CAD build for the part. Positions are in the model's coordinates, mm. Coordinates: 2 decimals unless noted, no trailing zeros.
1) Saw through at A-A, the plane z = -5. Give the number of separate pieces and of enclosed holes in the cut face, and give its area (3 significant figures).
2) Wall check: line 1 along Y through (x, z) = (0, -11); line 2 along X through (y, z) = (52.5, -1); line 3 along Z through (x, y) = (66.5, 3). Give the ranges that are in metal, low to high.
3) Pin check, flat tips, straight feed: pin 1 Ø1 at (x, z) = (14.5, -12.5) entering from -Y; pin 2 Ø5 at (y, z) = (-6, -10) entering from +X; pin 3 Ø3 at (x, z) = (46, -1) entering from -Y; pin 4 Ø11 at (x, y) = (0, 0) entering from +Z. Stop position of each tip, or through.
```python
from build123d import *

# Parameters (mm, degrees)
CUT_EXTRUDE1_DEPTH      = 117.550418275
CUT_EXTRUDE1_DEPTH_BACK = 117.550418275


with BuildPart() as part:
    # Sketch1 → Revolve1 (revolve)
    with BuildSketch(Plane(origin=(0, 0, 0), x_dir=(0, 0, -1), z_dir=(1, 0, 0)), mode=Mode.PRIVATE) as revolve1_sk:
        Polygon((-14, 80), (14, 80), (14, 65), (10, 65), (10, 13), (18, 13), (18, 6), (-18, 6), (-18, 13), (-10, 13), (-10, 65), (-14, 65), align=None)
    revolve(revolve1_sk.sketch.rotate(Axis((0, 0, 21.009226083), (0, 0, -1)), 90), axis=Axis((0, 0, 21.009226083), (0, 0, -1)))

    # Sketch2 → Cut-Extrude1 (cut, two sides: drawn at the far end of the back side and taken through both)
    with BuildSketch(Plane(origin=(0, 0, -10), x_dir=(-1, 0, 0), z_dir=(0, 0, -1)).offset(-CUT_EXTRUDE1_DEPTH_BACK)):
        with BuildLine():
            Line((0.637719681, 16.747637536), (7.842487003, 59.087331998))
            ThreePointArc((7.842487003, 59.087331998), (7.789998599, 59.614078882), (7.47597205, 60.040229838))
            ThreePointArc((7.47597205, 60.040229838), (-4.486988844, 63.647600818), (-15.699134285, 58.13277051))
            ThreePointArc((-15.699134285, 58.13277051), (-15.940556782, 57.654586316), (-15.900550292, 57.120409916))
            Line((-15.900550292, 57.120409916), (-1.288879604, 16.576347699))
            ThreePointArc((-1.288879604, 16.576347699), (-0.259550601, 15.919320899), (0.637719681, 16.747637536))
        make_face()
        with BuildLine():
            Line((7.394463789, 15.040344235), (31.197451444, 50.789136914))
            ThreePointArc((31.197451444, 50.789136914), (31.36374816, 51.291693094), (31.250201842, 51.80872747))
            ThreePointArc((31.250201842, 51.80872747), (21.78874322, 59.969999397), (9.302855115, 59.492341617))
            ThreePointArc((9.302855115, 59.492341617), (8.887809655, 59.153693995), (8.707088287, 58.649427466))
            Line((8.707088287, 58.649427466), (5.56475791, 15.667481708))
            ThreePointArc((5.56475791, 15.667481708), (6.23785987, 14.648592036), (7.394463789, 15.040344235))
        make_face()
        with BuildLine():
            Line((12.872637931, 10.732438778), (49.15809311, 33.709038652))
            ThreePointArc((49.15809311, 33.709038652), (49.514420733, 34.1005076), (49.620987836, 34.619025454))
            ThreePointArc((49.620987836, 34.619025454), (44.297003636, 45.92304027), (32.696296351, 50.565146389))
            ThreePointArc((32.696296351, 50.565146389), (32.17939306, 50.424590588), (31.809192199, 50.037426194))
            Line((31.809192199, 50.037426194), (11.456198227, 12.049565795))
            ThreePointArc((11.456198227, 12.049565795), (11.6566877, 10.844988532), (12.872637931, 10.732438778))
        make_face()
        with BuildLine():
            Line((16.12501603, 4.568797156), (58.618853889, 10.800341371))
            ThreePointArc((58.618853889, 10.800341371), (59.103600137, 11.013034549), (59.411854241, 11.443379433))
            ThreePointArc((59.411854241, 11.443379433), (59.145909698, 23.935570282), (50.436250912, 32.894777979))
            ThreePointArc((50.436250912, 32.894777979), (49.906867064, 32.976617376), (49.411197804, 32.773499358))
            Line((49.411197804, 32.773499358), (15.366757794, 6.348170489))
            ThreePointArc((15.366757794, 6.348170489), (15.05996833, 5.166187987), (16.12501603, 4.568797156))
        make_face()
        with BuildLine():
            Line((16.589232367, -2.384831001), (57.943882296, -13.975833051))
            ThreePointArc((57.943882296, -13.975833051), (58.473230137, -13.978692226), (58.929871308, -13.710930852))
            ThreePointArc((58.929871308, -13.710930852), (63.767950649, -2.190577255), (59.455319492, 9.536603618))
            ThreePointArc((59.455319492, 9.536603618), (59.004990363, 9.826687436), (58.469558421, 9.842736744))
            Line((58.469558421, 9.842736744), (16.620265336, -0.450881165))
            ThreePointArc((16.620265336, -0.450881165), (15.859243619, -1.405893394), (16.589232367, -2.384831001))
        make_face()
        with BuildLine():
            Line((14.185019719, -8.926100213), (47.24988705, -36.335458973))
            ThreePointArc((47.24988705, -36.335458973), (47.732307435, -36.553376123), (48.258378264, -36.494496632))
            ThreePointArc((48.258378264, -36.494496632), (57.36393362, -27.937954084), (58.194023196, -15.470536147))
            ThreePointArc((58.194023196, -15.470536147), (57.900614785, -15.022366034), (57.418001208, -14.789924471))
            Line((57.418001208, -14.789924471), (14.999978011, -7.17197137))
            ThreePointArc((14.999978011, -7.17197137), (13.91631161, -7.734883035), (14.185019719, -8.926100213))
        make_face()
        with BuildLine():
            Line((9.328088295, -13.923965606), (28.385957082, -52.412353941))
            ThreePointArc((28.385957082, -52.412353941), (28.738035143, -52.807649211), (29.242573206, -52.967832403))
            ThreePointArc((29.242573206, -52.967832403), (41.041171333, -48.854604843), (46.870451614, -37.802679666))
            ThreePointArc((46.870451614, -37.802679666), (46.7846969, -37.273915943), (46.43834996, -36.865273382))
            Line((46.43834996, -36.865273382), (10.786058217, -12.65296257))
            ThreePointArc((10.786058217, -12.65296257), (9.567122898, -12.726441131), (9.328088295, -13.923965606))
        make_face()
        with BuildLine():
            Line((2.858245661, -16.514250851), (4.613837255, -59.426676761))
            ThreePointArc((4.613837255, -59.426676761), (4.774695497, -59.931000008), (5.170461579, -60.282548753))
            ThreePointArc((5.170461579, -60.282548753), (17.622017675, -61.323850595), (27.442553143, -53.598396444))
            ThreePointArc((27.442553143, -53.598396444), (27.579279895, -53.080467163), (27.429086125, -52.566281616))
            Line((27.429086125, -52.566281616), (4.70713097, -15.946141593))
            ThreePointArc((4.70713097, -15.946141593), (3.563691723, -15.517481939), (2.858245661, -16.514250851))
        make_face()
        with BuildLine():
            Line((-4.105813613, -16.249072097), (-19.956056948, -56.165587294))
            ThreePointArc((-19.956056948, -56.165587294), (-20.014232376, -56.691736448), (-19.795669826, -57.173864775))
            ThreePointArc((-19.795669826, -57.173864775), (-8.84414293, -63.189645469), (3.269587926, -60.126463551))
            ThreePointArc((3.269587926, -60.126463551), (3.605154846, -59.708923389), (3.677084113, -59.178102208))
            Line((3.677084113, -59.178102208), (-2.185701986, -16.482087868))
            ThreePointArc((-2.185701986, -16.482087868), (-3.055934127, -15.625409147), (-4.105813613, -16.249072097))
        make_face()
        with BuildLine():
            Line((-10.359940414, -13.174281159), (-41.07536761, -43.192957537))
            ThreePointArc((-41.07536761, -43.192957537), (-41.342517649, -43.649956627), (-41.338950081, -44.179300168))
            ThreePointArc((-41.338950081, -44.179300168), (-33.781070876, -54.129376582), (-21.468718747, -56.258118879))
            ThreePointArc((-21.468718747, -56.258118879), (-20.992334227, -56.013164323), (-20.710719147, -55.557491313))
            Line((-20.710719147, -55.557491313), (-8.700607211, -14.168131416))
            ThreePointArc((-8.700607211, -14.168131416), (-9.147161204, -13.031561162), (-10.359940414, -13.174281159))
        make_face()
        with BuildLine():
            Line((-14.8227394, -7.821537324), (-55.092374054, -22.751873025))
            ThreePointArc((-55.092374054, -22.751873025), (-55.522306034, -23.060702758), (-55.734350314, -23.545733206))
            ThreePointArc((-55.734350314, -23.545733206), (-52.876944776, -35.709646734), (-42.494888911, -42.662234363))
            ThreePointArc((-42.494888911, -42.662234363), (-41.960058003, -42.632220281), (-41.517450915, -42.330485445))
            Line((-41.517450915, -42.330485445), (-13.711098407, -9.404376329))
            ThreePointArc((-13.711098407, -9.404376329), (-13.656761009, -8.184437864), (-14.8227394, -7.821537324))
        make_face()
        with BuildLine():
            Line((-16.722552084, -1.116378629), (-59.583408526, 1.623217027))
            ThreePointArc((-59.583408526, 1.623217027), (-60.101783302, 1.515956117), (-60.492775047, 1.159104933))
            ThreePointArc((-60.492775047, 1.159104933), (-62.829914552, -11.115394554), (-56.173306729, -21.689661952))
            ThreePointArc((-56.173306729, -21.689661952), (-55.672506555, -21.879778052), (-55.145438246, -21.784154084))
            Line((-55.145438246, -21.784154084), (-16.350816127, -3.014519138))
            ThreePointArc((-16.350816127, -3.014519138), (-15.804982768, -1.922150906), (-16.722552084, -1.116378629))
        make_face()
        with BuildLine():
            Line((-15.730883592, 5.781812073), (-53.771930365, 25.717638108))
            ThreePointArc((-53.771930365, 25.717638108), (-54.28911623, 25.830492408), (-54.791449415, 25.6635233))
            ThreePointArc((-54.791449415, 25.6635233), (-61.91902131, 15.400810325), (-60.138849494, 3.033250056))
            ThreePointArc((-60.138849494, 3.033250056), (-59.758672955, 2.655876574), (-59.238278324, 2.528855421))
            Line((-59.238278324, 2.528855421), (-16.163329196, 3.896575798))
            ThreePointArc((-16.163329196, 3.896575798), (-15.220379423, 4.672493406), (-15.730883592, 5.781812073))
        make_face()
        with BuildLine():
            Line((-12.019202417, 11.680274941), (-38.662796942, 45.365245923))
            ThreePointArc((-38.662796942, 45.365245923), (-39.08936776, 45.678701899), (-39.616184414, 45.730485342))
            ThreePointArc((-39.616184414, 45.730485342), (-50.301766767, 39.254075187), (-53.705838838, 27.231685572))
            ThreePointArc((-53.705838838, 27.231685572), (-53.512021911, 26.732306013), (-53.088281917, 26.40460285))
            Line((-53.088281917, 26.40460285), (-13.181055808, 10.133917379))
            ThreePointArc((-13.181055808, 10.133917379), (-12.004034203, 10.45922116), (-12.019202417, 11.680274941))
        make_face()
        with BuildLine():
            Line((-6.229291953, 15.55911216), (-16.868514687, 57.168790588))
            ThreePointArc((-16.868514687, 57.168790588), (-17.130712489, 57.628648854), (-17.590921227, 57.89023102))
            ThreePointArc((-17.590921227, 57.89023102), (-29.986879773, 56.319953837), (-37.986600745, 46.721515261))
            ThreePointArc((-37.986600745, 46.721515261), (-38.012656136, 46.186476887), (-37.758839274, 45.714754568))
            Line((-37.758839274, 45.714754568), (-7.919658125, 14.619012581))
            ThreePointArc((-7.919658125, 14.619012581), (-6.712082415, 14.437454556), (-6.229291953, 15.55911216))
        make_face()
    extrude(amount=CUT_EXTRUDE1_DEPTH + CUT_EXTRUDE1_DEPTH_BACK, mode=Mode.SUBTRACT)


solid = part.part
```
Data:
1. separate pieces: 1
1. enclosed holes: 16
1. area: 10,500 mm2
2. line 1: y = -80 to -65, -13 to -6, 6 to 13, 65 to 80
2. line 2: x = -60.36 to -30.87, -8.26 to -6.72, 14.24 to 15.67, 34.71 to 60.36
2. line 3: z = -14 to 14
3. pin 1: stops at y = -78.77
3. pin 2: stops at x = 79.92
3. pin 3: stops at y = -66.48
3. pin 4: passes through
